Input: dimensioned drawing with shaded views. Units: mm. Origin: part minimum x, y, z. A direction names the side the tool comes from. Round coordinates to 2 decimals unless told otherwise and drop trailing zeros. Order: outer loops, then holes, each group sorted by start corner. A loop starts at its lowest first (then second) coordinate and runs counter-clockwise, first axis right, second up.
Item 1: Mould query, pull axis Z, two halves, no side actions, for the marked faces 1, 2 and 3. Classes: released by +Z, released by -Z, zero draft, split by the parting line, or undercut.
Item 2: Cut plane A-A on z = 31.5. Output: boundary loops of the cut face in (x, y), then the cut area to 3 significant figures.
Item 3: Cut plane C-C on x = 10. Output: boundary loops of the cut face in (y, z).
Item 4: Cut plane D-D on z = 58. Output: boundary loops of the cut face in (x, y), then the cut area to 3 significant figures.
Item 5: Reachability of the marked faces 4, 5 and 6 from +Z, -Z, +X, -X, +Y, -Y: full face, straight path, thin tool, end or side. Return the list, or none.
Item 6: Line query: L1, parallel to X at y = 1, z = 31.5; L2, parallel to Z at x = 44, y = 18.75; L3, parallel to X at y = 2.4, z = 31.5. Output: solid intervals per line, ascending.
Item 7: Cut plane B-B on y = 13.5. Output: boundary loops of the cut face in (x, z).
Item 8: First-contact query: pin 1 (5 mm diameter, centred on x = 38, y = 17.5, fed in from -Z); pin 2 (4 mm diameter, centred on x = 50, z = 31.5, fed in from -Y); pin 3 (10 mm diameter, centred on x = 12, z = 48, fed in from +Y). Flat tips, straight axial feed; report the tip coordinate or a pass-through.
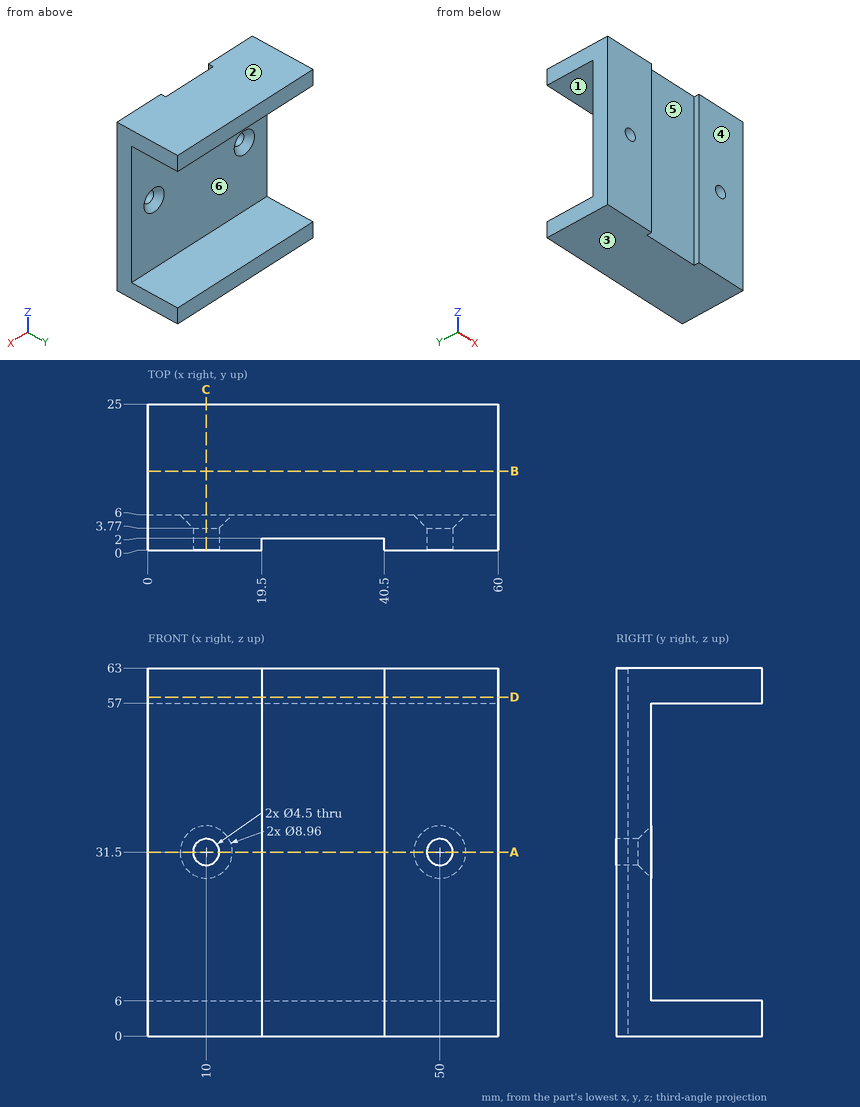
From the geometry:
1. face 1: undercut
1. face 2: released by +Z
1. face 3: released by -Z
2. outline: (0, 0) - (7.75, 0) - (7.75, 3.77) - (5.52, 6) - (0, 6) - close; (12.25, 0) - (19.5, 0) - (19.5, 2) - (40.5, 2) - (40.5, 0) - (47.75, 0) - (47.75, 3.77) - (45.52, 6) - (14.48, 6) - (12.25, 3.77) - close; (52.25, 0) - (60, 0) - (60, 6) - (54.48, 6) - (52.25, 3.77) - close
2. area: 254 mm2
3. outline: (0, 0) - (25, 0) - (25, 6) - (6, 6) - (6, 27.02) - (3.77, 29.25) - (0, 29.25) - close; (0, 33.75) - (3.77, 33.75) - (6, 35.98) - (6, 57) - (25, 57) - (25, 63) - (0, 63) - close
4. outline: (0, 0) - (19.5, 0) - (19.5, 2) - (40.5, 2) - (40.5, 0) - (60, 0) - (60, 25) - (0, 25) - close
4. area: 1,460 mm2
5. face 4: +Z, -Z, +X, -X, -Y
5. face 5: +Z, -Z, -Y
5. face 6: +X, -X, +Y
6. L1: x = 0 to 7.75, 12.25 to 19.5, 40.5 to 47.75, 52.25 to 60
6. L2: z = 0 to 6, 57 to 63
6. L3: x = 0 to 7.75, 12.25 to 47.75, 52.25 to 60
7. outline: (0, 0) - (60, 0) - (60, 6) - (0, 6) - close; (0, 57) - (60, 57) - (60, 63) - (0, 63) - close
8. pin 1: stops at z = 0
8. pin 2: passes through
8. pin 3: stops at y = 6
